Can you work these out from the drawing? Everything is in mm from the part's minimum corner. Round coordinates to 2 decimals unless told otherwise and drop trailing zeros. Loops run counter-clockwise (first coordinate to the right, second up) from the corner with the lowest first, then second, coordinate; pieces in that order, holes last. Notation, with made-up numbers: (27, 13) -> (52, 13) arc R22 ccw to (52, 21) -> close; hole circle Ø3 at (67, 72). An arc over 180 degrees is marked (long way). Answer as a JSON object with one key per item and string values.
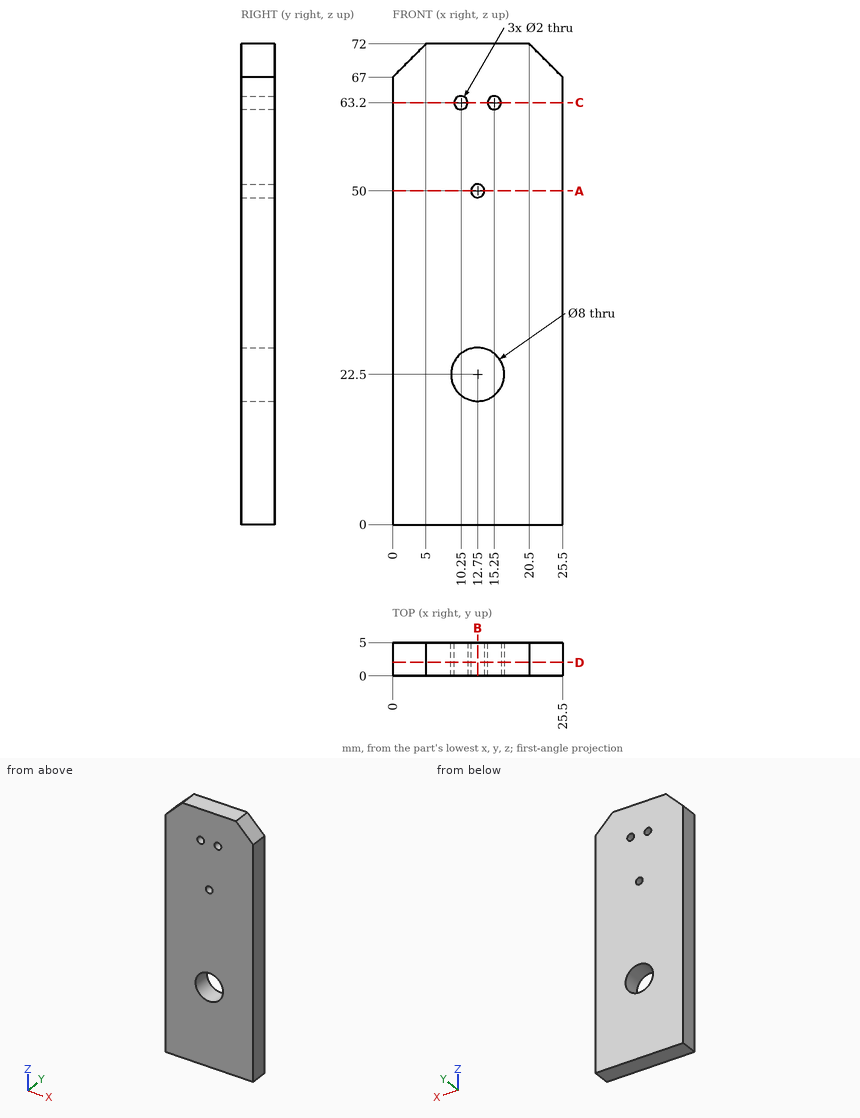
Q1. I want a section at C-C, the plane z = 63.2. Write out the boundary of the cut face in (x, y), then the cut area to 4 significant figures.
Determined:
{"outline": "(0, 0) -> (9.25, 0) -> (9.25, 5) -> (0, 5) -> close; (11.25, 0) -> (14.25, 0) -> (14.25, 5) -> (11.25, 5) -> close; (16.25, 0) -> (25.5, 0) -> (25.5, 5) -> (16.25, 5) -> close", "area": "107.5 mm²"}
Q2. I want a section at A-A, the plane z = 50. Write out the boundary of the cut face in (x, y), then the cut area to 4 significant figures.
Determined:
{"outline": "(0, 0) -> (11.75, 0) -> (11.75, 5) -> (0, 5) -> close; (13.75, 0) -> (25.5, 0) -> (25.5, 5) -> (13.75, 5) -> close", "area": "117.5 mm²"}
Q3. I'm going to push a flat-ended pin straight in: pin 1 (1.2 mm diameter, centred on x = 15.25, z = 63.2, fed in from +Y). Where does the tip first touch, or does it pass through?
Determined:
{"pin 1": "through"}
Q4. If I drill on L1, parallel to Z at x = 12.75, y = 4; L2, parallel to Z at x = 11, y = 4.2; L3, parallel to Z at x = 23, y = 1.1, over which ranges is the centre line in solid material (lowest first)? Write a range as [from, to].
Determined:
{"L1": "[0, 18.5], [26.5, 49], [51, 72]", "L2": "[0, 18.9], [26.1, 62.54], [63.86, 72]", "L3": "[0, 69.5]"}
Q5. I want a section at B-B, the plane x = 12.75. Write out the boundary of the cut face in (y, z).
Determined:
{"outline": "(0, 0) -> (5, 0) -> (5, 18.5) -> (0, 18.5) -> close; (0, 26.5) -> (5, 26.5) -> (5, 49) -> (0, 49) -> close; (0, 51) -> (5, 51) -> (5, 72) -> (0, 72) -> close"}
Q6. I want a section at D-D, the plane y = 2.05. Write out the boundary of the cut face in (x, z).
Determined:
{"outline": "(0, 0) -> (25.5, 0) -> (25.5, 67) -> (20.5, 72) -> (5, 72) -> (0, 67) -> close; hole circle Ø8 at (12.75, 22.5); hole circle Ø2 at (10.25, 63.2); hole circle Ø2 at (12.75, 50); hole circle Ø2 at (15.25, 63.2)"}
